Model file for the job. Use its own axes, mm. A direction names the side the tool comes from. Round coordinates to 2 decimals unless told otherwise and drop trailing zeros. Order: outer loops, then holes, each group sorted by start corner. A loop starts at its lowest first (then second) coordinate and runs counter-clockwise, first axis right, second up. Notation, with made-up numbers: M 9.5,-3.75 L 14.5,-3.75 A16 ccw 14.5,16.25 Z; hole C -5,42.5 d2. An arc over 180 degrees is marked long. Return JSON: item names as keys, results as strings. Group by question number.
Item 1: Slice it at B-B on y = -1. Write the cut outline in (x, z), then the cut area to 3 significant figures.
Item 2: Pin check, flat tip, straight feed: pin 1 Ø3 at (x, z) = (-30, 4.5) entering from -Y. Stop position of the tip, or through.
Item 3: Which spindle directions (+Z, -Z, +X, -X, +Y, -Y) get a long thin tool onto all of the face, cutting with end or side? Do faces 5 (the face through (44.722, 42.93, 1.449)), 6 (the face through (43.3, -43.1, 2.9)), 7 (the face through (45, 38, 9)). Say none if no direction does.
Item 4: Slice it at C-C on x = 13. Write the cut outline in (y, z), then the cut area to 3 significant figures.
Item 5: Pull direction X, two halves, no side cores. Call faces 1 (the face through (5.34, 32.03, 1)), 2 (the face through (1, 1, 2.032)), 3 (the face through (46.25, 44, 12)), 4 (the face through (-45, 38, 9)): pulls with the +X half, pulls with the -X half, needs draft (parallel to the pull), parting line crosses it, or undercut.
Item 6: Slice it at A-A on z = 17.5. Write the cut outline in (x, y).
Item 7: Probe line 1 along X through (y, z) = (-30.5, 1.25); line 2 along Z through (x, y) = (19.5, 1). List the from-to ranges inside material, lowest first.
from build123d import *

# Parameters (mm, degrees)
BOSS_EXTRUDE1_DEPTH     = 48
BOSS_EXTRUDE2_START     = 48
BOSS_EXTRUDE2_DEPTH     = 10
BOSS_EXTRUDE3_START     = -48
BOSS_EXTRUDE3_DEPTH     = 10
CONVERT_SOLID1_START    = -48
CONVERT_SOLID1_DEPTH    = 10
CONVERT_SOLID1_START_2  = 38
CONVERT_SOLID1_2_DEPTH  = 10
CONVERT_SOLID1_3_DEPTH  = 2.032
CONVERT_SOLID1_4_DEPTH  = 11.016
CONVERT_SOLID1_START_3  = 36.984
CONVERT_SOLID1_5_DEPTH  = 11.016
CUT_EXTRUDE1_DEPTH      = 70.243230716
CUT_EXTRUDE1_DEPTH_BACK = 70.243230716
SKETCH6_R               = 1.59
SKETCH7_R               = 1.5
CUT_EXTRUDE3_DEPTH      = 2.032


# Read off the part's stored shape, not the designer's step: Convert-Solid1
with BuildPart() as part:
    # Sketch1 → Boss-Extrude1 (new, symmetric)
    with BuildSketch(Plane(origin=(0, 0, 0), x_dir=(1, 0, 0), z_dir=(0, 1, 0))):
        Polygon((-44.218, 0), (-46.25, 0), (-46.25, -2.032), (-44.218, -2.032), (44.218, -2.032), (46.25, -2.032), (46.25, 0), (44.218, 0), align=None)
    extrude(amount=BOSS_EXTRUDE1_DEPTH, both=True)

    # Sketch1<3> → Boss-Extrude2 (add)
    with BuildSketch(Plane(origin=(0, 0, 0), x_dir=(1, 0, 0), z_dir=(0, 1, 0)).offset(BOSS_EXTRUDE2_START)):
        Polygon((-46.25, 0), (46.25, 0), (46.25, -18.75), (44.218, -18.75), (44.218, -2.032), (-44.218, -2.032), (-44.218, -18.75), (-46.25, -18.75), align=None)
    extrude(amount=-BOSS_EXTRUDE2_DEPTH)

    # Sketch1<4> → Boss-Extrude3 (add)
    with BuildSketch(Plane(origin=(0, 0, 0), x_dir=(1, 0, 0), z_dir=(0, 1, 0)).offset(BOSS_EXTRUDE3_START)):
        Polygon((-46.25, 0), (46.25, 0), (46.25, -18.75), (44.218, -18.75), (44.218, -2.032), (-44.218, -2.032), (-44.218, -18.75), (-46.25, -18.75), align=None)
    extrude(amount=BOSS_EXTRUDE3_DEPTH)

    # Convert-Solid1 outline → Convert-Solid1 (add)
    with BuildSketch(Plane(origin=(0, 0, 0), x_dir=(1, 0, 0), z_dir=(0, 1, 0)).offset(CONVERT_SOLID1_START)):
        with BuildLine():
            ThreePointArc((41.17, -2.032), (43.325261469, -2.924738531), (44.218, -5.08))
            Line((44.218, -5.08), (44.218, -2.032))
            Line((44.218, -2.032), (41.17, -2.032))
        make_face()
        with BuildLine():
            ThreePointArc((-44.218, -5.08), (-43.325261469, -2.924738531), (-41.17, -2.032))
            Line((-41.17, -2.032), (-44.218, -2.032))
            Line((-44.218, -2.032), (-44.218, -5.08))
        make_face()
    extrude(amount=CONVERT_SOLID1_DEPTH)

    # Convert-Solid1 2 outline → Convert-Solid1 2 (add)
    with BuildSketch(Plane(origin=(0, 0, 0), x_dir=(1, 0, 0), z_dir=(0, 1, 0)).offset(CONVERT_SOLID1_START_2)):
        with BuildLine():
            ThreePointArc((41.17, -2.032), (43.325261469, -2.924738531), (44.218, -5.08))
            Line((44.218, -5.08), (44.218, -2.032))
            Line((44.218, -2.032), (41.17, -2.032))
        make_face()
        with BuildLine():
            ThreePointArc((-44.218, -5.08), (-43.325261469, -2.924738531), (-41.17, -2.032))
            Line((-41.17, -2.032), (-44.218, -2.032))
            Line((-44.218, -2.032), (-44.218, -5.08))
        make_face()
    extrude(amount=CONVERT_SOLID1_2_DEPTH)

    # Convert-Solid1 3 outline → Convert-Solid1 3 (cut)
    with BuildSketch(Plane.XY):
        with BuildLine():
            ThreePointArc((39.138, -36.984), (38.63, -37.492), (39.138, -38))
            Line((39.138, -38), (46.25, -38))
            Line((46.25, -38), (46.25, -36.984))
            Line((46.25, -36.984), (39.138, -36.984))
        make_face()
        with BuildLine():
            Line((39.138, 36.984), (46.25, 36.984))
            Line((46.25, 36.984), (46.25, 38))
            Line((46.25, 38), (39.138, 38))
            ThreePointArc((39.138, 38), (38.63, 37.492), (39.138, 36.984))
        make_face()
        with BuildLine():
            Line((-46.25, -36.984), (-46.25, -38))
            Line((-46.25, -38), (-39.138, -38))
            ThreePointArc((-39.138, -38), (-38.63, -37.492), (-39.138, -36.984))
            Line((-39.138, -36.984), (-46.25, -36.984))
        make_face()
        with BuildLine():
            Line((-39.138, 38), (-46.25, 38))
            Line((-46.25, 38), (-46.25, 36.984))
            Line((-46.25, 36.984), (-39.138, 36.984))
            ThreePointArc((-39.138, 36.984), (-38.63, 37.492), (-39.138, 38))
        make_face()
    extrude(amount=CONVERT_SOLID1_3_DEPTH, mode=Mode.SUBTRACT)

    # Convert-Solid1 4 outline → Convert-Solid1 4 (cut)
    with BuildSketch(Plane(origin=(0, 0, 0), x_dir=(1, 0, 0), z_dir=(0, 1, 0)).offset(CONVERT_SOLID1_START)):
        with BuildLine():
            Line((46.25, -5.08), (46.25, 0))
            Line((46.25, 0), (41.17, 0))
            ThreePointArc((41.17, 0), (44.762102448, -1.487897552), (46.25, -5.08))
        make_face()
        with BuildLine():
            Line((-46.25, 0), (-46.25, -5.08))
            ThreePointArc((-46.25, -5.08), (-44.762102448, -1.487897552), (-41.17, 0))
            Line((-41.17, 0), (-46.25, 0))
        make_face()
    extrude(amount=CONVERT_SOLID1_4_DEPTH, mode=Mode.SUBTRACT)

    # Convert-Solid1 5 outline → Convert-Solid1 5 (cut)
    with BuildSketch(Plane(origin=(0, 0, 0), x_dir=(1, 0, 0), z_dir=(0, 1, 0)).offset(CONVERT_SOLID1_START_3)):
        with BuildLine():
            Line((46.25, -5.08), (46.25, 0))
            Line((46.25, 0), (41.17, 0))
            ThreePointArc((41.17, 0), (44.762102448, -1.487897552), (46.25, -5.08))
        make_face()
        with BuildLine():
            Line((-46.25, 0), (-46.25, -5.08))
            ThreePointArc((-46.25, -5.08), (-44.762102448, -1.487897552), (-41.17, 0))
            Line((-41.17, 0), (-46.25, 0))
        make_face()
    extrude(amount=CONVERT_SOLID1_5_DEPTH, mode=Mode.SUBTRACT)

    # Sketch6 → Cut-Extrude1 (cut, two sides: drawn at the far end of the back side and taken through both)
    with BuildSketch(Plane(origin=(0, 0, 0), x_dir=(0, 0, -1), z_dir=(1, 0, 0)).offset(-CUT_EXTRUDE1_DEPTH_BACK)):
        with Locations((-10.535, 42.865)):
            Circle(SKETCH6_R)
        with Locations((-7.995, -42.865)):
            Circle(SKETCH6_R)
    extrude(amount=CUT_EXTRUDE1_DEPTH + CUT_EXTRUDE1_DEPTH_BACK, mode=Mode.SUBTRACT)

    # Sketch7 → Cut-Extrude3 (cut)
    with BuildSketch(Plane(origin=(0, 0, 0), x_dir=(-1, 0, 0), z_dir=(0, 0, -1))):
        with Locations((-5.148, 30.54163056)):
            Circle(SKETCH7_R)
        with Locations((-5.148, -30.54163056)):
            Circle(SKETCH7_R)
    extrude(amount=-CUT_EXTRUDE3_DEPTH, mode=Mode.SUBTRACT)


solid = part.part
Output values:
{
 "1": {"outline": "M -46.25,0 L 46.25,0 L 46.25,2.03 L -46.25,2.03 Z", "area": "188 mm²"},
 "2": {"pin 1": "through"},
 "3": {"face 5": "-Z, +X, +Y", "face 6": "+Z, +Y, -Y", "face 7": "+Z, -Z, +X"},
 "4": {"outline": "M -48,0 L 48,0 L 48,2.03 L -48,2.03 Z", "area": "195 mm²"},
 "5": {"face 1": "undercut", "face 2": "undercut", "face 3": "pulls with the +X half", "face 4": "needs draft"},
 "6": {"outline": "M -46.25,-48 L -44.22,-48 L -44.22,-38 L -46.25,-38 Z; M -46.25,38 L -44.22,38 L -44.22,48 L -46.25,48 Z; M 44.22,-48 L 46.25,-48 L 46.25,-38 L 44.22,-38 Z; M 44.22,38 L 46.25,38 L 46.25,48 L 44.22,48 Z"},
 "7": {"line 1": "-46.25 to 3.65, 6.65 to 46.25", "line 2": "0 to 2.03"}
}
